Could you check a few things on this drawing? It's one solid part, dimensions in mm from its lowest x, y, z. A direction names the side the tool comes from. Round coordinates to 2 decimals unless told otherwise and drop trailing zeros. Order: outer loops, then holes, each group sorted by start corner. A loop starts at its lowest first (then second) coordinate and runs counter-clockwise, first axis right, second up.
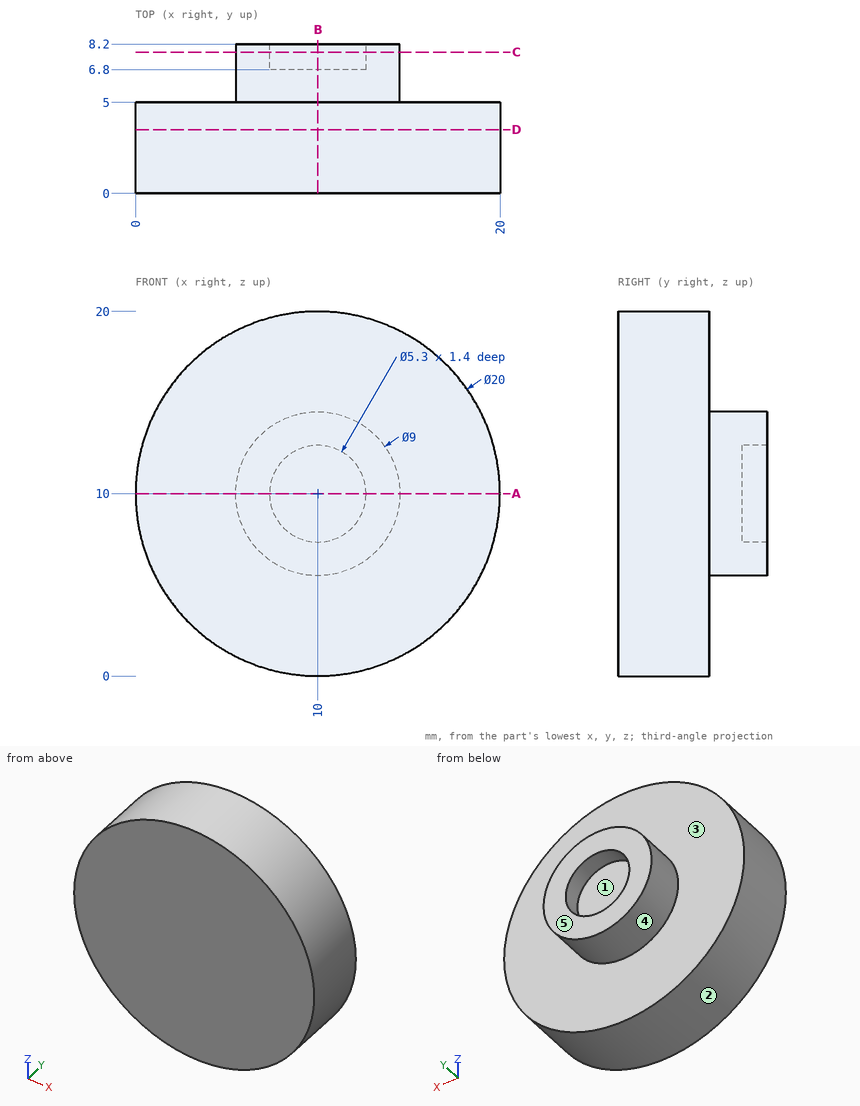
(1) I want a section at A-A, the plane z = 10. List the corners of the cut face in (x, y) for me.
(2) Please list where these lines run through material, in increasing order: probe 1 along Z at (x, y) = (10, 7.6); probe 2 along Y at (x, z) = (12.75, 4.25); probe 3 along Z at (x, y) = (11.25, 8).
(3) I want a section at C-C, the plane y = 7.75. List the corners of the cut face in (x, z) for me, plus the area to 3 significant figures.
(4) I want a section at B-B, the plane x = 10. List the corners of the cut face in (y, z) for me, plus the area to 3 significant figures.
(5) I want a section at D-D, the plane y = 3.5. List the corners of the cut face in (x, z) for me.
(6) If we mould it in two halves opening along Z, with no side actions, what happens to the marked faces 1, 2 and 3? For each: pulls with the +Z half, pulls with the -Z half, needs draft (parallel to the pull), parting line crosses it, or undercut.
(7) I'm going to push flat-ended pins straight in: pin 1 Ø8 at (x, z) = (4.5, 4.5) entering from -Y; pin 2 Ø1 at (x, y) = (6.5, 4) entering from +Z; pin 3 Ø2.5 at (x, z) = (11, 10) entering from +Y; pin 4 Ø4 at (y, z) = (6, 13) entering from +X. Where does each tip first touch, or does it pass through?
(8) On a 3-axis mill with a long thin cutter (end or side, diameter ignored), from which of +Z, -Z, +X, -X, +Y, -Y can I reach the whole of each face in a straight line? I mean the marked faces 4 and 5. Say none if no direction works.
Ans:
1. outline: (0, 0) - (20, 0) - (20, 5) - (14.5, 5) - (14.5, 8.2) - (12.65, 8.2) - (12.65, 6.8) - (7.35, 6.8) - (7.35, 8.2) - (5.5, 8.2) - (5.5, 5) - (0, 5) - close
2. probe 1: z = 5.5 to 7.35, 12.65 to 14.5
2. probe 2: y = 0 to 5
2. probe 3: z = 5.68 to 7.66, 12.34 to 14.32
3. outline: circle Ø9 at (10, 10); hole circle Ø5.3 at (10, 10)
3. area: 41.6 mm2
4. outline: (0, 0) - (5, 0) - (5, 5.5) - (8.2, 5.5) - (8.2, 7.35) - (6.8, 7.35) - (6.8, 12.65) - (8.2, 12.65) - (8.2, 14.5) - (5, 14.5) - (5, 20) - (0, 20) - close
4. area: 121 mm2
5. outline: circle Ø20 at (10, 10)
6. face 1: undercut
6. face 2: parting line crosses it
6. face 3: needs draft
7. pin 1: stops at y = 0
7. pin 2: stops at z = 19.54
7. pin 3: stops at y = 6.8
7. pin 4: stops at x = 19.92
8. face 4: +Y
8. face 5: +Z, -Z, +X, -X, +Y
